Check sheet for the modelled part. Datum: model origin and axes. Units: mm. Round coordinates to 2 decimals unless told otherwise and drop trailing zeros. Write each loop counter-clockwise with the first axis right and the second up, starting at its lowest first coordinate (ties: lowest second). Pieces come first, ordered by that corner, then holes. Notation, with made-up numbers: (-26.5, 60.5) -> (14.5, 60.5) arc R24 ccw to (14.5, 81.5) -> close; hole circle Ø2 at (19, 6.5). An arc over 180 degrees is marked (long way). One line per item, written item: value.
from build123d import *

# Parameters (mm, degrees)
F2_R    = 1.8
F3_SIZE = 1


with BuildPart() as f1:
    # F0 (on Right) → F1 (revolve)
    with BuildSketch(Plane.YZ):
        with BuildLine():
            Line((-10, 40.5), (-10, 7))
            Line((-10, 7), (10, 7))
            Line((10, 7), (10, 37.098887))
            Line((10, 37.098887), (-5.317889, 37.5))
            Line((-5.317889, 37.5), (-6.03756, 40.885786))
            ThreePointArc((-6.03756, 40.885786), (-8.193805, 42.490588), (-10, 40.5))
        make_face()
    revolve(axis=Axis((0, -1.591644, 0), (0, 1, 0)))

    # F2
    f2_edges = [f1.edges().sort_by_distance(p)[0] for p in [
        (0, -5.317889, -37.5),
    ]]
    fillet(f2_edges, radius=F2_R)

    # F3
    f3_edges = [f1.edges().sort_by_distance(p)[0] for p in [
        (0, 10, -37.098887),
    ]]
    chamfer(f3_edges, length=F3_SIZE)


solid = f1.part
Item 1: Depth check by flat-ended pin: pin 1 (22.5 mm diameter, centred on x = 0, z = 0, fed in from -Y); pin 2 (3 mm diameter, centred on x = 24.5, y = 4.5, fed in from -Z); pin 3 (5 mm diameter, centred on x = 31, y = 6, fed in from +Z); pin 4 (10 mm diameter, centred on x = 11.5, y = -6.5, fed in from -Z). Enter the tip coordinate at first touch or a pass-through.
Result set:
pin 1: y = -10
pin 2: z = -29.29
pin 3: z = 23.92
pin 4: z = -41.97
Item 2: Material ranges on line 1 along Z through (x, y) = (-4, 2); line 2 along X through (y, z) = (-5, 0); line 3 along X through (y, z) = (5.25, 0), recorded low to high.
Result set:
line 1: -37.09 to -5.74, 5.74 to 37.09
line 2: -37.88 to -7, 7 to 37.88
line 3: -37.22 to -7, 7 to 37.22
Item 3: Sectioned sample at A-A (y = 2.25). Enter the section's corners in (x, z), then the cut area to 3 significant figures.
Result set:
outline: circle Ø74.6 at (0, 0); hole circle Ø14 at (0, 0)
area: 4,220 mm^2
Item 4: Release check for a two-part mould opening along X. For faces 1 (the cylindrical face through (-2.681, 0.14, 6.466)), 2 (the flat face through (-8, -10, -1)), 3 (the conical face through (11.19, 3.89, 35.54)) record: pulls with the +X half, pulls with the -X half, needs draft (parallel to the pull), parting line crosses it, or undercut.
Result set:
face 1: undercut
face 2: needs draft
face 3: parting line crosses it
